Verification items for the finished model (mm, model axes). Round coordinates to 2 decimals unless told otherwise and drop trailing zeros. Order: outer loops, then holes, each group sorted by start corner. A loop starts at its lowest first (then second) coordinate and runs counter-clockwise, first axis right, second up. Notation, with made-up numbers: (16.5, 79) -> (64.5, 79) arc R14 cw to (64.5, 101) -> close; hole circle Ø10 at (76.5, 6). An arc over 180 degrees is marked (long way). Return JSON: item names as keys, results as strings. Group by question number.
Item 1: Sectioned sample at B-B on x = -42. Record the cut outline in (y, z), plus the area to 3 significant figures.
Item 2: Scan lines: probe 1 along Y at (x, z) = (-19, 127.5); probe 2 along Z at (x, y) = (-43, -15); probe 3 along X at (y, z) = (-7, 29). Record each from-to range of solid material in increasing order. Write a range as from..to.
Item 3: Depth check by flat-ended pin: pin 1 Ø7 at (x, y) = (-39.53, -7.94) entering from -Z; pin 2 Ø5 at (x, y) = (-9, -7) entering from -Z; pin 3 Ø6 at (y, z) = (-13.5, 53.5) entering from +X; pin 4 Ø2 at (x, z) = (-20, 115) entering from -Y. Enter the tip coordinate at first touch or a pass-through.
Item 4: Sectioned sample at D-D on y = -10.75. Record the cut outline in (x, z), plus the area to 3 significant figures.
Item 5: Sectioned sample at A-A on y = -4.25. Record the cut outline in (x, z), plus the area to 3 significant figures.
```python
from build123d import *

# Parameters (mm, degrees)
F0_R     = 5.953125
F1_DEPTH = 177.8
F3_R     = 7.9375
F4_DEPTH = 31.75


with BuildPart() as f1:
    # F0 (on Top) → F1 (new body)
    with BuildSketch(Plane.XY):
        with BuildLine():
            Line((0, -6.35), (0, 0))
            Line((0, 0), (-39.5271299333, 0))
            ThreePointArc((-39.5271299333, 0), (-44.5472457189, -14.0858610621), (-31.75, -6.35))
            Line((-31.75, -6.35), (0, -6.35))
        make_face()
        with Locations((-39.5271299333, -7.9375)):
            Circle(F0_R, mode=Mode.SUBTRACT)
    extrude(amount=F1_DEPTH)

    # F3 (on mid) → F4 (cut, symmetric)
    with BuildSketch(Plane.XY.offset(88.9)):
        with Locations((-39.5271299333, -7.9375)):
            Circle(F3_R)
    extrude(amount=F4_DEPTH, both=True, mode=Mode.SUBTRACT)


solid = f1.part
```
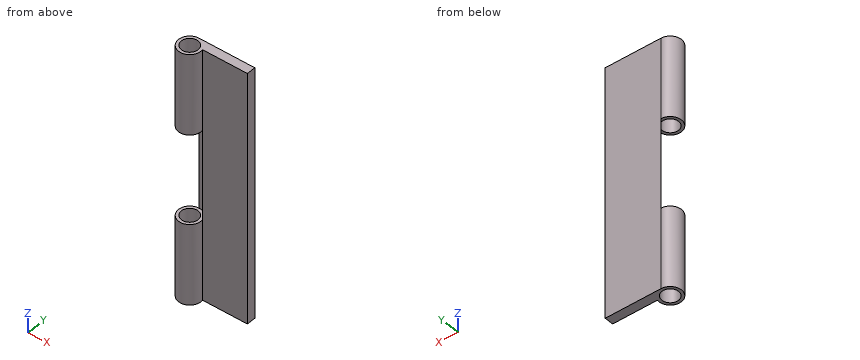
Recorded:
{
 "1": {"outline": "(-15.48, 0) -> (-13.35, 0) -> (-13.35, 57.15) -> (-15.48, 57.15) -> close; (-15.48, 120.65) -> (-13.35, 120.65) -> (-13.35, 177.8) -> (-15.48, 177.8) -> close; (-2.52, 0) -> (-0.4, 0) -> (-0.4, 57.15) -> (-2.52, 57.15) -> close; (-2.52, 120.65) -> (-0.4, 120.65) -> (-0.4, 177.8) -> (-2.52, 177.8) -> close", "area": "486 mm²"},
 "2": {"probe 1": "-6.35..0", "probe 2": "0..57.15, 120.65..177.8", "probe 3": "-47.41..-45.41, -33.65..-31.65"},
 "3": {"pin 1": "through", "pin 2": "z = 0", "pin 3": "x = -32.01", "pin 4": "y = -6.35"},
 "4": {"outline": "(-46.95, 0) -> (-44.77, 0) -> (-44.77, 57.15) -> (-46.95, 57.15) -> close; (-46.95, 120.65) -> (-44.77, 120.65) -> (-44.77, 177.8) -> (-46.95, 177.8) -> close; (-34.28, 0) -> (-32.1, 0) -> (-32.1, 57.15) -> (-34.28, 57.15) -> close; (-34.28, 120.65) -> (-32.1, 120.65) -> (-32.1, 177.8) -> (-34.28, 177.8) -> close", "area": "497 mm²"},
 "5": {"outline": "(-46.56, 0) -> (-44.2, 0) -> (-44.2, 57.15) -> (-46.56, 57.15) -> close; (-46.56, 120.65) -> (-44.2, 120.65) -> (-44.2, 177.8) -> (-46.56, 177.8) -> close; (-34.85, 0) -> (0, 0) -> (0, 177.8) -> (-34.85, 177.8) -> (-34.85, 120.65) -> (-32.5, 120.65) -> (-32.5, 57.15) -> (-34.85, 57.15) -> close", "area": "6,320 mm²"}
}
